The drawing under review shows one solid part. Ordinate dimensions are in mm from its lowest x, y, z. Give positions to 0.01 mm unless a question says otherwise; leave off trailing zeros. Order: outer loops, then holes, each group sorted by start corner. A loop starts at its lowest first (then second) coordinate and runs counter-clockwise, first axis right, second up. Notation, with made-up numbers: M -31.75,76 L -4.75,76 A19 cw -4.75,107 Z; hole C 47.25,-39.5 d9. An arc over 180 degrees is marked long. Put each result on its own line as item: value. Start each with the question number.
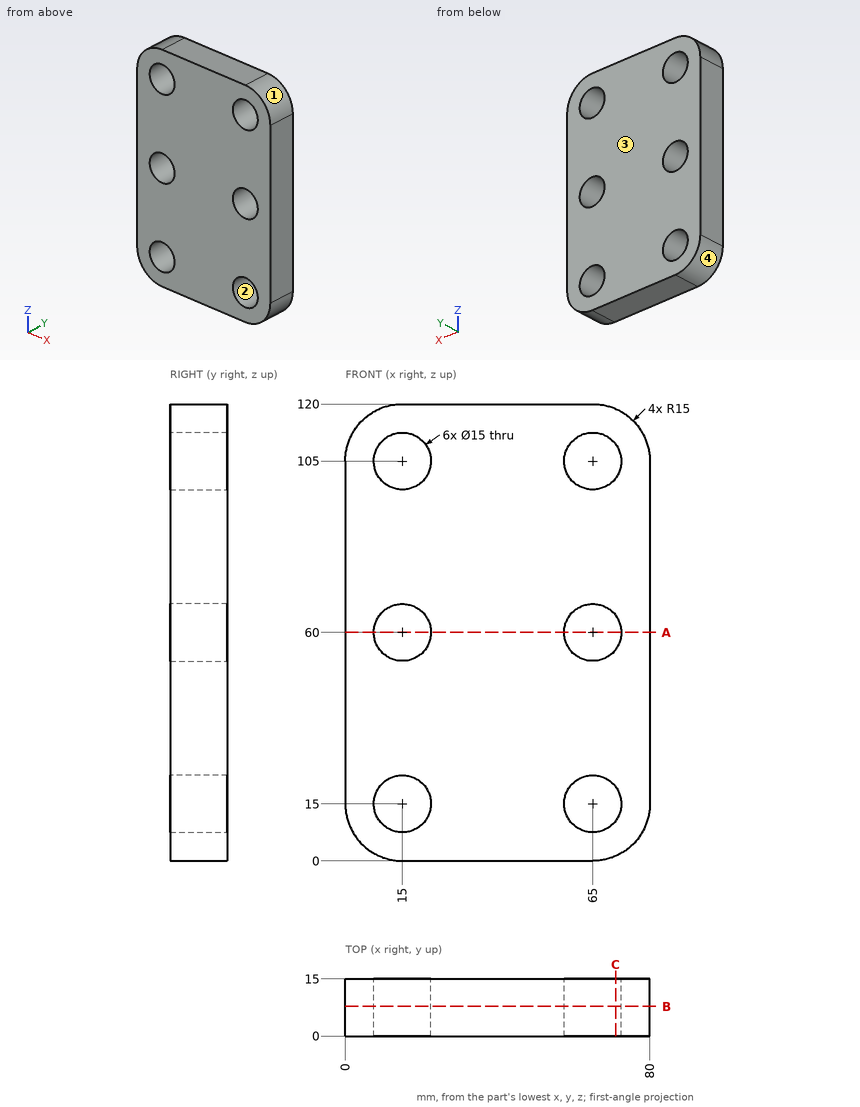
1. To check wall thickness, follow probe 1 along X at (y, z) = (11, 60); probe 2 along Z at (x, y) = (12.5, 12.25); probe 3 along X at (y, z) = (9.25, 108). State the ranges of each line that lie inside material, in increasing order.
2. The part is to be moulded in two halves that separate along X. For the marked faces 1, 2, 3 and 4, say which applies: +X half, -X half, draft (parallel to the pull), parting line (faces both ways), or undercut.
3. Consider section A-A on z = 60. Give the boundary of the cut face in (x, y).
4. Consider section C-C on x = 71. Give the boundary of the cut face in (y, z).
5. Consider section B-B on y = 7.75. Give the boundary of the cut face in (x, z).
6. Insertion check: pin 1 (13.5 mm diameter, centred on x = 15, z = 105, fed in from -Y). The pin has a flat end and moves straight along its axis. Give the tip position at first contact, or say it passes through.
Returned:
1. probe 1: x = 0 to 7.5, 22.5 to 57.5, 72.5 to 80
1. probe 2: z = 0.21 to 7.93, 22.07 to 52.93, 67.07 to 97.93, 112.07 to 119.79
1. probe 3: x = 0.3 to 8.13, 21.87 to 58.13, 71.87 to 79.7
2. face 1: +X half
2. face 2: undercut
2. face 3: draft
2. face 4: -X half
3. outline: M 0,0 L 7.5,0 L 7.5,15 L 0,15 Z; M 22.5,0 L 57.5,0 L 57.5,15 L 22.5,15 Z; M 72.5,0 L 80,0 L 80,15 L 72.5,15 Z
4. outline: M 0,1.25 L 15,1.25 L 15,10.5 L 0,10.5 Z; M 0,19.5 L 15,19.5 L 15,55.5 L 0,55.5 Z; M 0,64.5 L 15,64.5 L 15,100.5 L 0,100.5 Z; M 0,109.5 L 15,109.5 L 15,118.75 L 0,118.75 Z
5. outline: M 0,15 A15 ccw 15,0 L 65,0 A15 ccw 80,15 L 80,105 A15 ccw 65,120 L 15,120 A15 ccw 0,105 Z; hole C 15,15 d15; hole C 15,60 d15; hole C 15,105 d15; hole C 65,15 d15; hole C 65,60 d15; hole C 65,105 d15
6. pin 1: passes through
